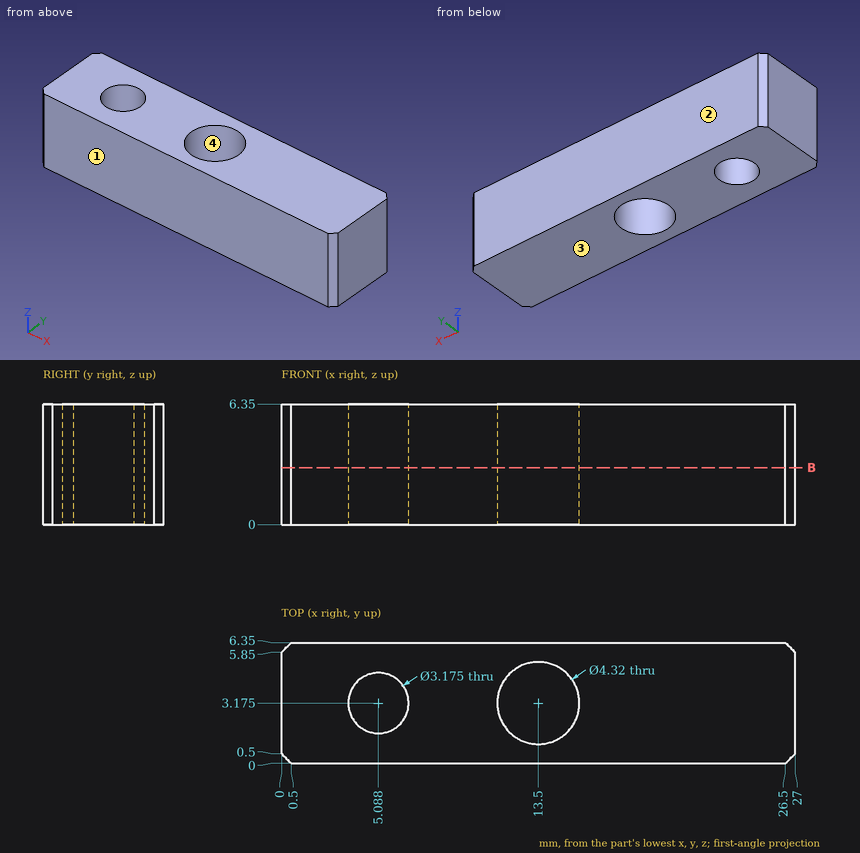
Design review of the part shown in the three views and the two pictorial views. Dimensions are in mm from the part's minimum x, y and z. Give positions to 0.01 mm unless a question says otherwise; leave off trailing zeros. Write each question's results on one line, items separated by ' | '. Start each with the question number.
Q1. Add section B-B on z = 3. State how many separate pieces and enclosed holes the cut face has, and give its area (3 significant figures).
Q2. Wall thickness on L1, parallel to X at y = 1.75, z = 1 (1 decimal); L2, parallel to X at y = 4.25, z = 1.5 (1 decimal); L3, parallel to Y at x = 15, z = 1.25: over which ranges is each line inside the solid? List them lowest first. Write a range as from..to.
Q3. Mouldability with a two-part tool opening along Y and no side actions: class the marked faces 1, 2, 3 and 4 as +Y half, -Y half, draft (parallel to the pull), parting line (faces both ways), or undercut.
Found:
1) separate pieces: 1 | enclosed holes: 2 | area: 148 mm2
2) L1: x = 0..4.4, 5.8..11.9, 15.1..27 | L2: x = 0..3.9, 6.3..11.6, 15.4..27 | L3: y = 0..1.62, 4.73..6.35
3) face 1: -Y half | face 2: +Y half | face 3: draft | face 4: undercut
